```python
from build123d import *

# Parameters (mm, degrees)
SKETCH1_W           = 121
SKETCH1_H           = 66
BOSS_EXTRUDE1_DEPTH = 4
SKETCH2_W           = 28
SKETCH2_H           = 28
SKETCH2_W_2         = 15
SKETCH2_H_2         = 12.5
CUT_EXTRUDE1_DEPTH  = 5
SKETCH3_W           = 5
SKETCH3_H           = 2
CUT_EXTRUDE2_DEPTH  = 5
SKETCH4_W           = 3.5
SKETCH4_H           = 13.5
CUT_EXTRUDE3_DEPTH  = 5


with BuildPart() as part:
    # Sketch1 → Boss-Extrude1 (new body)
    with BuildSketch(Plane(origin=(0, 0, 0), x_dir=(1, 0, 0), z_dir=(0, 1, 0))):
        with Locations((60.5, -33)):
            Rectangle(SKETCH1_W, SKETCH1_H)
    extrude(amount=BOSS_EXTRUDE1_DEPTH)

    # Sketch2 → Cut-Extrude1 (cut, through all)
    with BuildSketch(Plane(origin=(0, 4, 0), x_dir=(1, 0, 0), z_dir=(0, 1, 0))):
        with Locations((80.25, -33)):
            Rectangle(SKETCH2_W, SKETCH2_H)
        with Locations((46, -17)):
            Rectangle(SKETCH2_W_2, SKETCH2_H_2)
        with Locations((46, -49)):
            Rectangle(SKETCH2_W_2, SKETCH2_H_2)
    extrude(amount=-CUT_EXTRUDE1_DEPTH, mode=Mode.SUBTRACT)

    # Sketch3 → Cut-Extrude2 (cut, through all)
    with BuildSketch(Plane.XZ):
        with Locations((105, 49)):
            Rectangle(SKETCH3_W, SKETCH3_H)
        with Locations((105, 17)):
            Rectangle(SKETCH3_W, SKETCH3_H)
    extrude(amount=-CUT_EXTRUDE2_DEPTH, mode=Mode.SUBTRACT)

    # Sketch4 → Cut-Extrude3 (cut, through all)
    with BuildSketch(Plane(origin=(0, 4, 0), x_dir=(1, 0, 0), z_dir=(0, 1, 0))):
        with Locations((32.95, -49.395895757)):
            Rectangle(SKETCH4_W, SKETCH4_H)
        with Locations((32.95, -17.399625311)):
            Rectangle(SKETCH4_W, SKETCH4_H)
    extrude(amount=-CUT_EXTRUDE3_DEPTH, mode=Mode.SUBTRACT)


solid = part.part
```
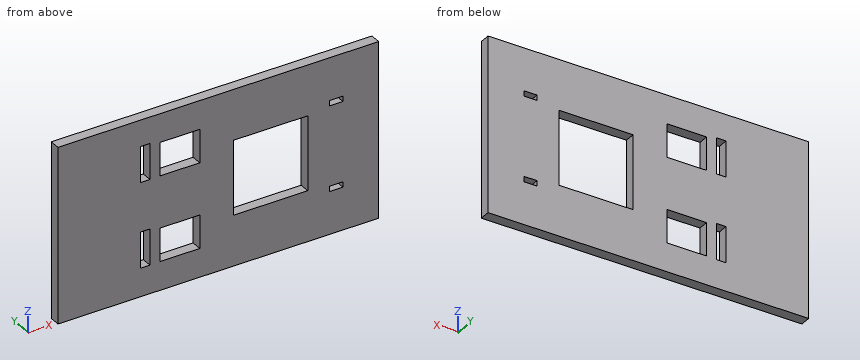
Check sheet for the modelled part. Datum: model origin and axes. Units: mm. Round coordinates to 2 decimals unless told otherwise and drop trailing zeros. Order: outer loops, then holes, each group sorted by start corner. A loop starts at its lowest first (then second) coordinate and runs counter-clockwise, first axis right, second up.
1) Section check D-D (z = 54). Record the boundary of the cut face in (x, y).
2) Go/stop test with a flat-tipped pin: pin 1 Ø1 at (y, z) = (2.5, 49.5) entering from -X. Record where the tip stops, or that it passes through.
3) Section check B-B (z = 44). Record the boundary of the cut face in (x, y).
4) Section check C-C (y = 2.6). Give the number of separate pieces and of enclosed holes in the cut face, and give its area (3 significant figures).
5) Section check A-A (x = 42.5). Record the boundary of the cut face in (y, z), and give its area (3 significant figures).
6) Scan lines: line 1 (Z direction, x = 39.5, y = 0.9); line 2 (Z direction, x = 106.5, y = 2.35); line 3 (Z direction, x = 76, y = 1.65). Record each from-to range of solid material in increasing order.
Result:
1. outline: (0, 0) - (31.2, 0) - (31.2, 4) - (0, 4) - close; (34.7, 0) - (38.5, 0) - (38.5, 4) - (34.7, 4) - close; (53.5, 0) - (121, 0) - (121, 4) - (53.5, 4) - close
2. pin 1: stops at x = 0
3. outline: (0, 0) - (31.2, 0) - (31.2, 4) - (0, 4) - close; (34.7, 0) - (38.5, 0) - (38.5, 4) - (34.7, 4) - close; (53.5, 0) - (66.25, 0) - (66.25, 4) - (53.5, 4) - close; (94.25, 0) - (121, 0) - (121, 4) - (94.25, 4) - close
4. separate pieces: 1
4. enclosed holes: 7
4. area: 6,710 mm2
5. outline: (0, 0) - (4, 0) - (4, 10.75) - (0, 10.75) - close; (0, 23.25) - (4, 23.25) - (4, 42.75) - (0, 42.75) - close; (0, 55.25) - (4, 55.25) - (4, 66) - (0, 66) - close
5. area: 164 mm2
6. line 1: z = 0 to 10.75, 23.25 to 42.75, 55.25 to 66
6. line 2: z = 0 to 16, 18 to 48, 50 to 66
6. line 3: z = 0 to 19, 47 to 66
